from build123d import *

# Parameters (mm, degrees)
REVOLVE1_ANGLE                 = 180
FILLET1_R                      = 2.5
FILLET2_R                      = 2.5
CUT_EXTRUDE1_DEPTH             = 70
BOSS_EXTRUDE1_DEPTH            = 70
SKETCH7_W                      = 5
SKETCH7_H                      = 5
REVOLVE2_ANGLE                 = 4
F_3_0MM_DOWEL_HOLE2_AT_2_COUNT = 2
F_3_0MM_DOWEL_HOLE2_AT_2_PITCH = 59.592915104
FILLET3_R                      = 2
FILLET3_OF_MIRROR3_R           = 2


with BuildPart() as part:
    # Sketch1 → Revolve1 (revolve)
    with BuildSketch(Plane.XY):
        with BuildLine():
            Line((4.330127019, 50), (0, 47.5))
            ThreePointArc((0, 47.5), (-4.264235636, 55.691520443), (-13.420201433, 56.896926208))
            Line((-13.420201433, 56.896926208), (-15.13030215, 61.595389312))
            ThreePointArc((-15.13030215, 61.595389312), (-4.86969785, 61.595389312), (2.990381057, 55))
            Line((2.990381057, 55), (75, 55))
            Line((75, 55), (75, 50))
            Line((75, 50), (4.330127019, 50))
        make_face()
    revolve(axis=Axis((-156.553254438, 0, 0), (1, 0, 0)), revolution_arc=REVOLVE1_ANGLE)

    # Fillet1
    fillet1_edges = [part.edges().sort_by_distance(p)[0] for p in [
        (4.330127019, 0, 50),
    ]]
    fillet(fillet1_edges, radius=FILLET1_R)

    # Fillet2
    fillet2_edges = [part.edges().sort_by_distance(p)[0] for p in [
        (-15.13030215, 0, 61.595389312),
        (-13.420201433, 0, 56.896926208),
    ]]
    fillet(fillet2_edges, radius=FILLET2_R - 0.0001)  # a hair under: the kernel refuses the full size

    # Sketch3 → Cut-Extrude1 (cut)
    with BuildSketch(Plane(origin=(75, 0, 0), x_dir=(0, 0, -1), z_dir=(1, 0, 0))):
        Polygon((0, 54), (0, 51), (-0.5, 51.5), (-0.5, 53.5), align=None)
    extrude(amount=-CUT_EXTRUDE1_DEPTH, mode=Mode.SUBTRACT)

    # Sketch5 → Boss-Extrude1 (add)
    with BuildSketch(Plane(origin=(75, 0, 0), x_dir=(0, 0, -1), z_dir=(1, 0, 0))):
        Polygon((0, -51.05), (0, -53.95), (0.5, -53.45), (0.5, -51.55), align=None)
    extrude(amount=-BOSS_EXTRUDE1_DEPTH)

    # Sketch7 → Revolve2 (revolve)
    with BuildSketch(Plane(origin=(0, 0, 0), x_dir=(-1, 0, 0), z_dir=(0, 0, -1))):
        with Locations((-69.608609025, 57.5)):
            Rectangle(SKETCH7_W, SKETCH7_H)
        with Locations((-10.015693921, 57.5)):
            Rectangle(SKETCH7_W, SKETCH7_H)
    revolve2 = revolve(axis=Axis((75, 0, 0), (1, 0, 0)), revolution_arc=REVOLVE2_ANGLE)

    # Sketch11 → Ø3.0mm Dowel Hole2 (revolve, cut)
    with BuildSketch(Plane(origin=(69.608609025, 57.5, 0), x_dir=(0, 1, 0), z_dir=(1, 0, 0))):
        Polygon((0, 0), (0, 45.991420021), (1.65, 45), (1.65, 0), align=None)
    f_3_0mm_dowel_hole2 = revolve(axis=Axis((69.608609025, 57.5, -6.35), (0, 0, 1)), mode=Mode.SUBTRACT)

    # Ø3.0mm Dowel Hole2 at 2: Ø3.0mm Dowel Hole2 ×2
    with Locations(*[(-i * F_3_0MM_DOWEL_HOLE2_AT_2_PITCH, 0, 0) for i in range(1, F_3_0MM_DOWEL_HOLE2_AT_2_COUNT)]):
        add(f_3_0mm_dowel_hole2, mode=Mode.SUBTRACT)

    # Fillet3
    fillet3_edges = [part.edges().sort_by_distance(p)[0] for p in [
        (72.108609025, 54.966495486, 1.919472319),
        (67.108609025, 54.966495486, 1.919472319),
        (67.108609025, 59.963449621, 2.093969802),
        (72.108609025, 59.963449621, 2.093969802),
        (7.515693921, 54.966495486, 1.919472319),
        (7.515693921, 59.963449621, 2.093969802),
        (12.515693921, 59.963449621, 2.093969802),
        (12.515693921, 54.966495486, 1.919472319),
    ]]
    fillet(fillet3_edges, radius=FILLET3_R)

    # Mirror3: Revolve2, Ø3.0mm Dowel Hole2 across plane
    add(revolve2.mirror(Plane.ZX))
    add(f_3_0mm_dowel_hole2.mirror(Plane.ZX), mode=Mode.SUBTRACT)

    # Mirror3 copy 1 sketch → Mirror3 copy 1 (revolve, cut)
    with BuildSketch(Plane(origin=(10.015693921, -57.5, 0), x_dir=(0, -1, 0), z_dir=(1, 0, 0))):
        Polygon((0, 0), (0, -45.991420021), (1.65, -45), (1.65, 0), align=None)
    revolve(axis=Axis((10.015693921, -57.5, -6.35), (0, 0, -1)), mode=Mode.SUBTRACT)

    # Fillet3 of Mirror3
    fillet3_of_mirror3_edges = [part.edges().sort_by_distance(p)[0] for p in [
        (72.108609025, -54.966495486, 1.919472319),
        (67.108609025, -54.966495486, 1.919472319),
        (67.108609025, -59.963449621, 2.093969802),
        (72.108609025, -59.963449621, 2.093969802),
        (7.515693921, -54.966495486, 1.919472319),
        (7.515693921, -59.963449621, 2.093969802),
        (12.515693921, -59.963449621, 2.093969802),
        (12.515693921, -54.966495486, 1.919472319),
    ]]
    fillet(fillet3_of_mirror3_edges, radius=FILLET3_OF_MIRROR3_R)


solid = part.part
Part model, mm, in its own coordinate system. A direction names the side the tool comes from. Coordinates: 2 decimals unless noted, no trailing zeros. Loops run counter-clockwise (first coordinate to the right, second up) from the corner with the lowest first, then second, coordinate; pieces in that order, holes last. Notation, with made-up numbers: M 21.5,45.25 L 32.5,45.25 A35 cw 32.5,82.25 Z; hole C 89.25,6 d1. An arc over 180 degrees is marked long. Use a Markdown table: item, result. Add a question column.
Q1. Pin check, flat tips, straight feed: P1, Ø4.5, axis at x = 10.02, y = -57.5, coming from the +Z side; P2, Ø1.3, axis at y = 57.5, z = 2, coming from the +X side; P3, Ø4, axis at x = 4, y = -20, coming from the -Z side; P4, Ø3, axis at x = 10.02, y = 57.5, coming from the -Z side. Stop position of each tip, or through.
Q2. Mould opens along X. For faces 1 (the flat face through (75, -4, 50)), 2 (the flat face through (20.6, 54.5, 0)), 3 (the cylindrical face through (68.493, -56.284, 2.039)) say: +X half, -X half, draft (parallel to the pull), parting line (faces both ways), or undercut.
Q3. Which spindle directions (+Z, -Z, +X, -X, +Y, -Y) get a long thin tool onto all of the face, cutting with end or side? Do faces 4 (the cylindrical face through (39.51, 1.099, 49.988)), 5 (the cylindrical face through (9.94, -55.85, 2.04)), 6 (the flat face through (10.037, 55.524, 3.883)). Say none if no direction does.
Q4. Probe L1, parallel to X at y = 57.5, z = 3.05; L2, parallel to X at y = -57.5, z = 2.85; L3, parallel to Y at x = 34, z = 4.5. List the from-to ranges inside material, lowest first.
Q5. Cut at A-A (x = 49.5). Write the cut outline in (y, z), and give its area (3 significant figures).
Worked out:
| question | item | result |
|---|---|---|
| 1 | P1 | stops at z = 4.18 |
| 1 | P2 | stops at x = 72.11 |
| 1 | P3 | stops at z = 44.05 |
| 1 | P4 | passes through |
| 2 | face 1 | +X half |
| 2 | face 2 | draft |
| 2 | face 3 | undercut |
| 3 | face 4 | -Z, +X |
| 3 | face 5 | +Z, -Z |
| 3 | face 6 | +Z, +X |
| 4 | L1 | x = -12.86 to 1.11, 7.52 to 8.37, 11.67 to 12.52, 67.11 to 67.96, 71.26 to 72.11 |
| 4 | L2 | x = -12.84 to 1.12, 7.52 to 8.37, 11.67 to 12.52, 67.11 to 67.96, 71.26 to 72.11 |
| 4 | L3 | y = -54.82 to -49.8, 49.8 to 54.82 |
| 5 | outline | M -55,0 L -53.95,0 L -53.45,-0.5 L -51.55,-0.5 L -51.05,0 L -50,0 A50 cw 50,0 L 51,0 L 51.5,0.5 L 53.5,0.5 L 54,0 L 55,0 A55 ccw Z |
| 5 | area | 825 mm2 |
